from build123d import *

# Parameters (mm, degrees)
BOSS_EXTRU_1_DEPTH                                = 59.2
BOSS_EXTRU_2_DEPTH                                = 1.5
BOSS_EXTRU_3_DEPTH                                = 44.45
ESQUISSE5_W                                       = 98
ESQUISSE5_H                                       = 50
ENL_V_MAT_EXTRU_1_DEPTH                           = 79.75
NERVURE3_REACH                                    = 219.919
ESQUISSE7_WALL_W                                  = 531.966109146
ESQUISSE7_WALL_H                                  = 10
ESQUISSE8_W                                       = 12.7
ESQUISSE8_H                                       = 12.7
ENL_V_MAT_EXTRU_2_DEPTH                           = 79.75
FRAISAGE_POUR_VIS_T_TE_FRAIS_E_BOMB_E_D           = 5.1054
FRAISAGE_POUR_VIS_T_TE_FRAIS_E_BOMB_E_CSINK_D     = 9.779
FRAISAGE_POUR_VIS_T_TE_FRAIS_E_BOMB_E_CSINK_ANGLE = 82
ENL_VEMENT_START                                  = 1.582341914
ENL_VEMENT_DE_MATI_RE_BALAYAGE2_OUTLINE_R         = 6.35
ENL_VEMENT_DE_MATI_RE_BALAYAGE2_DEPTH             = 71.529963189
ENL_VEMENT_START_2                                = -14.345570266
ENL_VEMENT_DE_MATI_RE_BALAYAGE3_OUTLINE_R         = 6.35
ENL_VEMENT_DE_MATI_RE_BALAYAGE3_DEPTH             = 71.529963189
ESQUISSE26_R                                      = 6.35
ENL_V_MAT_EXTRU_4_DEPTH                           = 3.175
NERVURE4_REACH                                    = 258.559
ESQUISSE27_WALL_W                                 = 609.246066174
ESQUISSE27_WALL_H                                 = 2.5
ESQUISSE29_R                                      = 3.5
ENL_V_MAT_EXTRU_7_DEPTH                           = 257.559080586
ESQUISSE28_R                                      = 5.55625
ENL_V_MAT_EXTRU_6_DEPTH                           = 47
ESQUISSE30_R                                      = 3.175
LETTRE_O_DEPTH                                    = 1
ESQUISSE31_W                                      = 1
ESQUISSE31_H                                      = 6.35
LETTRE_I_DEPTH                                    = 1
LETTRE_D_DEPTH                                    = 1
LETTRE_A_DEPTH                                    = 1
LETTRE_R_DEPTH                                    = 1
BOSS_EXTRU_5_REACH                                = 258.559
BOSS_EXTRU_6_DEPTH                                = 94.127905
BOSS_EXTRU_7_DEPTH                                = 2.5
ESQUISSE38_W                                      = 2.5
ESQUISSE38_H                                      = 2.446117838
BOSS_EXTRU_8_DEPTH                                = 94.127905
ENL_V_MAT_EXTRU_13_REACH                          = 263.075
BOSS_EXTRU_9_REACH                                = 245.841
ESQUISSE40_W                                      = 2.5
ESQUISSE40_H                                      = 105.15
ENL_V_MAT_EXTRU_14_REACH                          = 258.559


# Read off the part's stored shape, not the designer's step: Enlèvement de matière-Balayage2, Enlèvement de matière-Balayage3
with BuildPart() as part:
    # Esquisse2 → Boss.-Extru.1 (new body)
    with BuildSketch(Plane.XY):
        Polygon((0, 0), (98, 0), (98, 50), (211.579865137, 100), (-113.579865137, 100), (0, 50), align=None)
    extrude(amount=BOSS_EXTRU_1_DEPTH)

    # Esquisse3 → Boss.-Extru.2 (add)
    with BuildSketch(Plane.XY.offset(59.2)):
        Polygon((0, 0), (98, 0), (98, 50), (211.579865137, 100), (168.51775825, 100), (92.873568069, 66.7), (5.126431931, 66.7), (-70.51775825, 100), (-113.579865137, 100), (0, 50), align=None)
    extrude(amount=BOSS_EXTRU_2_DEPTH)

    # Esquisse4 → Boss.-Extru.3 (add)
    with BuildSketch(Plane.XY.offset(60.7)):
        Polygon((0, 0), (98, 0), (98, 50), (211.579865137, 100), (-113.579865137, 100), (0, 50), align=None)
    extrude(amount=BOSS_EXTRU_3_DEPTH)

    # Esquisse5 → Enlèv. mat.-Extru.1 (cut)
    with BuildSketch(Plane.XY.offset(105.15)):
        with Locations((49, 25)):
            Rectangle(ESQUISSE5_W, ESQUISSE5_H)
    extrude(amount=-ENL_V_MAT_EXTRU_1_DEPTH, mode=Mode.SUBTRACT)

    # Esquisse7 wall → Nervure3 (add, up to next)
    with BuildSketch(Plane(origin=(49, 25, 65.275), x_dir=(0, -0.531192105031, -0.847251407525), z_dir=(0, 0.847251407525, -0.531192105031)), mode=Mode.PRIVATE) as nervure3_sk1:
        Rectangle(ESQUISSE7_WALL_W, ESQUISSE7_WALL_H)
    nervure3_tool1 = extrude(nervure3_sk1.sketch, amount=NERVURE3_REACH, mode=Mode.PRIVATE) - part.part
    add(nervure3_tool1.solids().sort_by_distance((49, 25, 65.275))[0])

    # Esquisse8 → Enlèv. mat.-Extru.2 (cut)
    with BuildSketch(Plane.XY.offset(105.15)):
        with Locations((-8.15, 93.65)):
            Rectangle(ESQUISSE8_W, ESQUISSE8_H)
    enl_v_mat_extru_2 = extrude(amount=-ENL_V_MAT_EXTRU_2_DEPTH, mode=Mode.SUBTRACT)

    # Symétrie1: Enlèv. mat.-Extru.2 across plane
    add(enl_v_mat_extru_2.mirror(Plane(origin=(49, 0, 0), x_dir=(0, 0, 1), z_dir=(1, 0, 0))), mode=Mode.SUBTRACT)

    # Fraisage pour vis à tête fraisée bombée #101 (through all)
    with Locations(Plane.XY.offset(25.4)):
        with Locations((22, 25), (76, 25), (106.15, 93.65), (-8.15, 93.65)):
            CounterSinkHole(FRAISAGE_POUR_VIS_T_TE_FRAIS_E_BOMB_E_D / 2, FRAISAGE_POUR_VIS_T_TE_FRAIS_E_BOMB_E_CSINK_D / 2, counter_sink_angle=FRAISAGE_POUR_VIS_T_TE_FRAIS_E_BOMB_E_CSINK_ANGLE)

    # Enlèvement de matière-Balayage2 outline → Enlèvement de matière-Balayage2 (cut)
    with BuildSketch(Plane(origin=(0, 0, 0), x_dir=(0.8002544678430299, -0.3970882953901229, 0.44934805258444765), z_dir=(0.5996605595645498, 0.5299192642332058, -0.5996605595645498)).offset(ENL_VEMENT_START)):
        with Locations((6.44062437, -61.833135415)):
            Circle(ENL_VEMENT_DE_MATI_RE_BALAYAGE2_OUTLINE_R)
    extrude(amount=ENL_VEMENT_DE_MATI_RE_BALAYAGE2_DEPTH, mode=Mode.SUBTRACT)

    # Enlèvement de matière-Balayage3 outline → Enlèvement de matière-Balayage3 (cut)
    with BuildSketch(Plane(origin=(0, 0, 0), x_dir=(0.8002544678430281, 0.39708829539012125, -0.4493480525844523), z_dir=(0.5996605595645522, -0.5299192642332002, 0.5996605595645522)).offset(ENL_VEMENT_START_2)):
        with Locations((71.984313478, 61.833135415)):
            Circle(ENL_VEMENT_DE_MATI_RE_BALAYAGE3_OUTLINE_R)
    extrude(amount=ENL_VEMENT_DE_MATI_RE_BALAYAGE3_DEPTH, mode=Mode.SUBTRACT)

    # Esquisse26 → Enlèv. mat.-Extru.4 (cut)
    with BuildSketch(Plane(origin=(0, 0, 0), x_dir=(-1, 0, 0), z_dir=(0, 0, -1))):
        with Locations((-49, 82.52)):
            Circle(ESQUISSE26_R)
    extrude(amount=-ENL_V_MAT_EXTRU_4_DEPTH, mode=Mode.SUBTRACT)

    # Esquisse27 wall → Nervure4 (add, up to next)
    with BuildSketch(Plane(origin=(0, 25, 65.275), x_dir=(0, 0.531192105031, 0.847251407525), z_dir=(0, 0.847251407525, -0.531192105031)), mode=Mode.PRIVATE) as nervure4_sk1:
        with Locations((0, 1.25)):
            Rectangle(ESQUISSE27_WALL_W, ESQUISSE27_WALL_H)
    nervure4_tool1 = extrude(nervure4_sk1.sketch, amount=NERVURE4_REACH, mode=Mode.PRIVATE) - part.part
    nervure4 = nervure4_tool1.solids().sort_by_distance((0, 25, 65.275))[0]
    add(nervure4)

    # Symétrie5: Nervure4 across plane
    add(nervure4.mirror(Plane.ZY.offset(-49)))

    # Esquisse29 → Enlèv. mat.-Extru.7 (cut, through all)
    with BuildSketch(Plane(origin=(0, 100, 0), x_dir=(1, 0, 0), z_dir=(0, 1, 0))):
        with Locations(Location((80.75, -82.925, 0), (0, 0, 180))):
            Circle(ESQUISSE29_R)
        with Locations(Location((17.25, -82.925, 0), (0, 0, 180))):
            Circle(ESQUISSE29_R)
    extrude(amount=-ENL_V_MAT_EXTRU_7_DEPTH, mode=Mode.SUBTRACT)

    # Esquisse28 → Enlèv. mat.-Extru.6 (cut)
    with BuildSketch(Plane.XZ.offset(-50)):
        with Locations(Location((17.25, 82.925, 0), (0, 0, 270))):
            Circle(ESQUISSE28_R)
        with Locations(Location((80.75, 82.925, 0), (0, 0, 270))):
            Circle(ESQUISSE28_R)
    extrude(amount=-ENL_V_MAT_EXTRU_6_DEPTH, mode=Mode.SUBTRACT)

    # Esquisse30 → Lettre_O (cut)
    with BuildSketch(Plane(origin=(0, 100, 0), x_dir=(1, 0, 0), z_dir=(0, 1, 0))):
        with Locations(Location((91.625, -95.625, 0), (0, 0, 180))):
            Circle(ESQUISSE30_R)
    extrude(amount=-LETTRE_O_DEPTH, mode=Mode.SUBTRACT)

    # Esquisse31 → Lettre_I (cut)
    with BuildSketch(Plane(origin=(0, 100, 0), x_dir=(1, 0, 0), z_dir=(0, 1, 0))):
        with Locations((86.95, -95.625)):
            Rectangle(ESQUISSE31_W, ESQUISSE31_H)
    extrude(amount=-LETTRE_I_DEPTH, mode=Mode.SUBTRACT)

    # Esquisse32 → Lettre_D (cut)
    with BuildSketch(Plane(origin=(0, 100, 0), x_dir=(1, 0, 0), z_dir=(0, 1, 0))):
        with BuildLine():
            Line((82.275, -92.45), (82.275, -98.8))
            ThreePointArc((82.275, -98.8), (85.45, -95.625), (82.275, -92.45))
        make_face()
    extrude(amount=-LETTRE_D_DEPTH, mode=Mode.SUBTRACT)

    # Esquisse33 → Lettre_A (cut)
    with BuildSketch(Plane(origin=(0, 100, 0), x_dir=(1, 0, 0), z_dir=(0, 1, 0))):
        Polygon((77.629166667, -98.8), (78.629166667, -98.8), (79.202083333, -96.05), (79.702083333, -96.05), (80.275, -98.8), (81.275, -98.8), (79.952083333, -92.45), (78.952083333, -92.45), align=None)
    extrude(amount=-LETTRE_A_DEPTH, mode=Mode.SUBTRACT)

    # Esquisse34 → Lettre_R (cut)
    with BuildSketch(Plane(origin=(0, 100, 0), x_dir=(1, 0, 0), z_dir=(0, 1, 0))):
        with BuildLine():
            Line((73.593632761, -98.8), (73.593632761, -92.863864698))
            ThreePointArc((73.593632761, -92.863864698), (76.218088657, -93.289201214), (75.393480286, -95.816789182))
            Line((75.393480286, -95.816789182), (76.629166667, -98.8))
            Line((76.629166667, -98.8), (75.629166667, -98.8))
            Line((75.629166667, -98.8), (74.593632761, -96.3))
            Line((74.593632761, -96.3), (74.593632761, -98.8))
            Line((74.593632761, -98.8), (73.593632761, -98.8))
        make_face()
    extrude(amount=-LETTRE_R_DEPTH, mode=Mode.SUBTRACT)

    # Boss.-Extru.5: up to this face of the body (flat: up to its plane)
    boss_extru_5_end = Plane(part.part.faces().sort_by_distance((98, 30.090642155, 36.697287119))[0])
    # Esquisse35 → Boss.-Extru.5 (add, up to the picked face)
    with BuildSketch(Plane.ZY, mode=Mode.PRIVATE) as boss_extru_5_sk1:
        Polygon((25.4, 0), (28.385893417, -4.7625), (0, -4.7625), (0, 0), align=None)
    boss_extru_5_tool1 = split(extrude(boss_extru_5_sk1.sketch, amount=-BOSS_EXTRU_5_REACH, mode=Mode.PRIVATE), bisect_by=boss_extru_5_end, keep=Keep.BOTH, mode=Mode.PRIVATE)
    add(boss_extru_5_tool1.solids().sort_by(Axis((0, -2.425315, 13.460287), (1, 0, 0)))[0])

    # Esquisse36 → Boss.-Extru.6 (add)
    with BuildSketch(Plane(origin=(0, 11.43135277, 18.233007668), x_dir=(1, 0, 0), z_dir=(0, 0.5311921050311518, 0.8472514075246933))):
        Polygon((50.67, -13.492279468), (50.67, -16.667279468), (54, -16.667279468), (54, -19.113397306), (44, -19.113397306), (44, -16.667279468), (47.33, -16.667279468), (47.33, -13.492279468), align=None)
    extrude(amount=BOSS_EXTRU_6_DEPTH)

    # Esquisse37 → Boss.-Extru.7 (add)
    with BuildSketch(Plane(origin=(98, 0, 0), x_dir=(0, 0, -1), z_dir=(1, 0, 0))):
        Polygon((0, 50), (0, -4.7625), (-28.385893417, -4.7625), (-115.732080917, 50), align=None)
    boss_extru_7 = extrude(amount=BOSS_EXTRU_7_DEPTH)

    # Esquisse38 → Boss.-Extru.8 (add)
    with BuildSketch(Plane(origin=(0, 11.43135277, 18.233007668), x_dir=(1, 0, 0), z_dir=(0, 0.5311921050311518, 0.8472514075246933))):
        with Locations((96.75, -17.890338387)):
            Rectangle(ESQUISSE38_W, ESQUISSE38_H)
    boss_extru_8 = extrude(amount=BOSS_EXTRU_8_DEPTH)

    # Esquisse39 → Enlèv. mat.-Extru.13 (cut, up to next)
    with BuildSketch(Plane.ZY.offset(-98), mode=Mode.PRIVATE) as enl_v_mat_extru_13_sk1:
        Polygon((108.135893417, 45.2375), (105.15, 50), (115.732080917, 50), align=None)
    enl_v_mat_extru_13_tool1 = extrude(enl_v_mat_extru_13_sk1.sketch, amount=-ENL_V_MAT_EXTRU_13_REACH, mode=Mode.PRIVATE) & part.part
    enl_v_mat_extru_13 = enl_v_mat_extru_13_tool1.solids().sort_by_distance((98, 48.4125, 109.672658))[0]
    add(enl_v_mat_extru_13, mode=Mode.SUBTRACT)

    # Esquisse40 → Boss.-Extru.9 (add, up to next)
    with BuildSketch(Plane(origin=(0, 50, 0), x_dir=(1, 0, 0), z_dir=(0, 1, 0)), mode=Mode.PRIVATE) as boss_extru_9_sk1:
        with Locations((99.25, -52.575)):
            Rectangle(ESQUISSE40_W, ESQUISSE40_H)
    boss_extru_9_tool1 = extrude(boss_extru_9_sk1.sketch, amount=BOSS_EXTRU_9_REACH, mode=Mode.PRIVATE) - part.part
    boss_extru_9 = boss_extru_9_tool1.solids().sort_by_distance((99.25, 50, 52.575))[0]
    add(boss_extru_9)

    # Symétrie6: Boss.-Extru.7, Boss.-Extru.8, Enlèv. mat.-Extru.13, Boss.-Extru.9 across plane
    add(boss_extru_7.mirror(Plane.ZY.offset(-49)))
    add(boss_extru_8.mirror(Plane.ZY.offset(-49)))
    add(enl_v_mat_extru_13.mirror(Plane.ZY.offset(-49)), mode=Mode.SUBTRACT)
    add(boss_extru_9.mirror(Plane.ZY.offset(-49)))

    # Esquisse41 → Enlèv. mat.-Extru.14 (cut, up to next)
    with BuildSketch(Plane.XY.offset(105.15), mode=Mode.PRIVATE) as enl_v_mat_extru_14_sk1:
        Polygon((112.5, 100), (112.5, 56.38317363), (211.579865137, 100), align=None)
    enl_v_mat_extru_14_tool1 = extrude(enl_v_mat_extru_14_sk1.sketch, amount=-ENL_V_MAT_EXTRU_14_REACH, mode=Mode.PRIVATE) & part.part
    # Esquisse41 → Enlèv. mat.-Extru.14 (cut, up to next)
    with BuildSketch(Plane.XY.offset(105.15), mode=Mode.PRIVATE) as enl_v_mat_extru_14_sk2:
        Polygon((-14.5, 100), (-14.5, 56.38317363), (-113.579865137, 100), align=None)
    enl_v_mat_extru_14_tool2 = extrude(enl_v_mat_extru_14_sk2.sketch, amount=-ENL_V_MAT_EXTRU_14_REACH, mode=Mode.PRIVATE) & part.part
    add(enl_v_mat_extru_14_tool1.solids().sort_by_distance((145.526622, 85.461058, 105.15))[0], mode=Mode.SUBTRACT)
    add(enl_v_mat_extru_14_tool2.solids().sort_by_distance((-47.526622, 85.461058, 105.15))[0], mode=Mode.SUBTRACT)


solid = part.part
Geometry: final body of the model. Coordinates: model frame, mm. A direction names the side the tool comes from. Coordinates: 2 decimals unless noted, no trailing zeros. Loops run counter-clockwise (first coordinate to the right, second up) from the corner with the lowest first, then second, coordinate; pieces in that order, holes last. Notation, with made-up numbers: (-16.75, 64) - (-5.75, 64) arc R15 cw to (-5.75, 83) - close; hole circle Ø5 at (16.5, 9.25). An arc over 180 degrees is marked (long way). One line per question, with ' | ' between items. Start each with the question number.
(1) Ray query, L1, parallel to X at y = 15.5, z = 59; L2, parallel to Z at x = 47.5, y = 94.5; L3, parallel to X at y = 66, z = 78.5. Return the intervals inside material, ascending. Write a range as from..to.
(2) Draft query along Z for faces 1 (the flat face through (49.07, 19.887, 67.703)), 2 (the flat face through (99.8, 94, 43)), 3 (the flat face through (52.31, 25.35, 65.83)), 4 (the flat face through (96.73, 21.96, 66.4)). Return one class per face: +Z half, -Z half, draft (parallel to the pull), parting line (faces both ways), or undercut.
(3) Cut plane C-C on y = 36. Output: boundary loops of the cut face in (x, z), and give its area (3 significant figures).
(4) Reachability of faces 5 (the cylindrical face through (88.597, 99.507, 96.579)), 6 (the flat face through (-8, 87.3, 83)), 7 (the flat face through (50.67, 23, 66)), 8 (the flat face through (106, 87.3, 83)), 9 (the cylindrical face through (77.369, 73.171, 87.334)) from +Z, -Z, +X, -X, +Y, -Y: full face, straight path, thin tool, end or side. Return the list, or none.
(5) First-contact query: pin 1 (6.5 mm diameter, centred on x = 105, y = 91, fed in from +Z); pin 2 (4 mm diameter, centred on x = 104.5, z = 40, fed in from +Y); pin 3 (16.5 mm diameter, centred on x = 29, y = 78.5, fed in from +Z). Flat tips, straight axial feed; report the tip coordinate or a pass-through.
(6) Cut plane A-A on y = 93.65. Count the separate pieces of the cut face and the enclosed holes in it, and give its area (3 significant figures).
(7) Cut plane B-B on x = 106.15. Output: boundary loops of the cut face in (y, z).
Here are the results:
1) L1: -2.5..2.5, 44..54, 95.5..100.5 | L2: 0..59.2, 60.7..105.15 | L3: -14.5..13.89, 20.61..77.39, 84.11..112.5
2) face 1: +Z half | face 2: draft | face 3: undercut | face 4: undercut
3) outline: (-2.5, 0) - (100.5, 0) - (100.5, 93.4) - (95.5, 93.4) - (95.5, 88.8) - (98, 88.8) - (98, 82.82) - (95.5, 82.82) - (95.5, 25.4) - (54, 25.4) - (54, 82.82) - (50.67, 82.82) - (50.67, 88.8) - (54, 88.8) - (54, 93.4) - (44, 93.4) - (44, 88.8) - (47.33, 88.8) - (47.33, 82.82) - (44, 82.82) - (44, 25.4) - (2.5, 25.4) - (2.5, 82.82) - (0, 82.82) - (0, 88.8) - (2.5, 88.8) - (2.5, 93.4) - (-2.5, 93.4) - close | area: 3,910 mm²
4) face 5: +Y | face 6: +Z, -X, +Y | face 7: none | face 8: +Z, +X, +Y | face 9: -Y
5) pin 1: z = 25.4 | pin 2: y = 87.3 | pin 3: z = 105.15
6) separate pieces: 4 | enclosed holes: 2 | area: 10,700 mm²
7) outline: (53.59, 0) - (91.1, 0) - (91.1, 22.71) - (88.76, 25.4) - (87.3, 25.4) - (87.3, 59.2) - (72.54, 59.2) - (72.54, 60.7) - (87.3, 60.7) - (87.3, 105.15) - (53.59, 105.15) - close; (96.2, 0) - (100, 0) - (100, 25.4) - (98.54, 25.4) - (96.2, 22.71) - close
